```python
from build123d import *

# Parameters (mm, degrees)
SKETCH1_R           = 1.5
SKETCH1_R_2         = 2
BOSS_EXTRUDE1_DEPTH = 2


with BuildPart() as part:
    # Sketch1 → Boss-Extrude1 (new body)
    with BuildSketch(Plane(origin=(0, 0, 0), x_dir=(1, 0, 0), z_dir=(0, 1, 0))):
        with BuildLine():
            Line((-93.5, -35.464771253), (-93.5, -12.5))
            Line((-93.5, -12.5), (-64.5, -12.5))
            Line((-64.5, -12.5), (-64.5, -76.418256981))
            ThreePointArc((-64.5, -76.418256981), (0, -100), (64.5, -76.418256981))
            Line((64.5, -76.418256981), (64.5, -12.5))
            Line((64.5, -12.5), (93.5, -12.5))
            Line((93.5, -12.5), (93.5, -35.464771253))
            ThreePointArc((93.5, -35.464771253), (0, 100), (-93.5, -35.464771253))
        make_face()
        with Locations((-50, -69)):
            Circle(SKETCH1_R, mode=Mode.SUBTRACT)
        with BuildLine():
            Line((-22, -67.5), (-16, -67.5))
            ThreePointArc((-16, -67.5), (-14.5, -69), (-16, -70.5))
            Line((-16, -70.5), (-22, -70.5))
            ThreePointArc((-22, -70.5), (-23.5, -69), (-22, -67.5))
        make_face(mode=Mode.SUBTRACT)
        with Locations((-50, -20)):
            Circle(SKETCH1_R, mode=Mode.SUBTRACT)
        with BuildLine():
            ThreePointArc((-16, -18.5), (-14.5, -20), (-16, -21.5))
            Line((-16, -21.5), (-22, -21.5))
            ThreePointArc((-22, -21.5), (-23.5, -20), (-22, -18.5))
            Line((-22, -18.5), (-16, -18.5))
        make_face(mode=Mode.SUBTRACT)
        with BuildLine():
            ThreePointArc((16, -70.5), (14.5, -69), (16, -67.5))
            Line((16, -67.5), (22, -67.5))
            ThreePointArc((22, -67.5), (23.5, -69), (22, -70.5))
            Line((22, -70.5), (16, -70.5))
        make_face(mode=Mode.SUBTRACT)
        with Locations((50, -69)):
            Circle(SKETCH1_R, mode=Mode.SUBTRACT)
        with BuildLine():
            Line((22, -21.5), (16, -21.5))
            ThreePointArc((16, -21.5), (14.5, -20), (16, -18.5))
            Line((16, -18.5), (22, -18.5))
            ThreePointArc((22, -18.5), (23.5, -20), (22, -21.5))
        make_face(mode=Mode.SUBTRACT)
        with Locations((50, -20)):
            Circle(SKETCH1_R, mode=Mode.SUBTRACT)
        with Locations((-60, 60)):
            Circle(SKETCH1_R_2, mode=Mode.SUBTRACT)
        with Locations((-20, 65)):
            Circle(SKETCH1_R_2, mode=Mode.SUBTRACT)
        with Locations((20, 65)):
            Circle(SKETCH1_R_2, mode=Mode.SUBTRACT)
        with Locations((60, 60)):
            Circle(SKETCH1_R_2, mode=Mode.SUBTRACT)
    extrude(amount=BOSS_EXTRUDE1_DEPTH)


solid = part.part
```
Could you check a few things on this model? Use its own coordinates, in mm. Coordinates: 2 decimals unless noted, no trailing zeros. Order: outer loops, then holes, each group sorted by start corner. A loop starts at its lowest first (then second) coordinate and runs counter-clockwise, first axis right, second up. Notation, with made-up numbers: M 85.5,-30 L 109.5,-30 A25 cw 109.5,1 Z; hole C 79.5,-35.5 d10. An arc over 180 degrees is marked long. Use one line per item in the form item = value. Start each with the question number.
1. We'd pull the mould along Z, two halves only. Please class faces 1 (the cylindrical face through (2.706, 0.986, -99.963)), 2 (the flat face through (-1, 0, -1)), 3 (the cylindrical face through (-0.981, 0.986, 99.995)): +Z half, -Z half, draft (parallel to the pull), parting line (faces both ways), or undercut.
2. Suppose I cut it at B-B on z = 30. Write out the boundary of the cut face in (x, y).
3. Suppose I cut it at A-A on y = 0.7. Count the separate pieces of the cut face and the enclosed holes in it, then the cut area to 3 significant figures.
4. Please list where these lines run through material, in increasing order: line 1 (X direction, y = 1.5, z = 69); line 2 (X direction, y = 0.5, z = -65); line 3 (X direction, y = 1.1, z = -60).
5. Suppose I cut it at D-D on z = -25.5. Write out the boundary of the cut face in (x, y).
6. For pin 1 (0.6 mm diameter, centred on x = 19.5, y = 1, fed in from -Z); pin 2 (6.5 mm diameter, centred on x = -60, z = -60, fed in from -Y); pin 3 (1 mm diameter, centred on y = 0.5, z = 26, fed in from +X), each with a flat end and sliding along its axis, tell me the tip position at first contact or that it passes through.
7. Suppose I cut it at C-C on x = 37.5. Write out the boundary of the cut face in (y, z).
Geometry says:
q1.face_1 = parting line
q1.face_2 = draft
q1.face_3 = +Z half
q2.outline = M -95.39,0 L -93.5,0 L -93.5,2 L -95.39,2 Z; M -64.5,0 L 64.5,0 L 64.5,2 L -64.5,2 Z; M 93.5,0 L 95.39,0 L 95.39,2 L 93.5,2 Z
q3.separate_pieces = 1
q3.enclosed_holes = 12
q3.area = 28,500 mm^2
q4.line_1 = -64.5 to -51.5, -48.5 to -23.5, -14.5 to 14.5, 23.5 to 48.5, 51.5 to 64.5
q4.line_2 = -75.99 to -22, -18 to 18, 22 to 75.99
q4.line_3 = -80 to -62, -58 to 58, 62 to 80
q5.outline = M -96.69,0 L 96.69,0 L 96.69,2 L -96.69,2 Z
q6.pin_1 = -98.14
q6.pin_2 = 0
q6.pin_3 = 96.69
q7.outline = M 0,-92.7 L 2,-92.7 L 2,92.7 L 0,92.7 Z
